Geometry check sheet. Reference: the model listing, model coordinates, mm. A direction names the side the tool comes from. Round coordinates to 2 decimals unless told otherwise and drop trailing zeros. Write each loop counter-clockwise with the first axis right and the second up, starting at its lowest first coordinate (ties: lowest second). Pieces come first, ordered by that corner, then holes. Notation, with made-up numbers: (24, 76.25) -> (74, 76.25) arc R25 ccw to (74, 97.25) -> close; hole circle Ø8 at (-8, 77). An arc over 180 degrees is marked (long way). One line per question, with ' | ' between items.
```python
from build123d import *

# Parameters (mm, degrees)
SKETCH_W           = 25.5
SKETCH_H           = 20.5
PAD_DEPTH          = 32
POCKET_DEPTH       = 20.501
SKETCH002_W        = 25.5
SKETCH002_H        = 2
POCKET001_DEPTH    = 2.1
SKETCH003_W        = 1.7
SKETCH003_H        = 9.5
POCKET002_DEPTH    = 12.5
SKETCH004_R        = 1.6
POCKET003_DEPTH    = 32.001
SKETCH005_R        = 3.6
POCKET004_DEPTH    = 2
SKETCH006_R        = 9
POCKET005_DEPTH    = 2
SKETCH007_R        = 3.6
POCKET006_DEPTH    = 19
SKETCH008_W        = 2.9999909846
SKETCH008_H        = 7.2
POCKET007_DEPTH    = 19
SKETCH009_W        = 2.9999856852
SKETCH009_H        = 3.2
POCKET008_DEPTH    = 7.5
SKETCH010_W        = 13
SKETCH010_H        = 15.5
PAD001_DEPTH       = 8.5
SKETCH011_W        = 16
SKETCH011_H        = 10
POCKET009_DEPTH    = 24
SKETCH012_W        = 4
SKETCH012_H        = 7.2
POCKET010_DEPTH    = 9
SKETCH013_W        = 1.5
SKETCH013_H        = 1.85
PAD002_DEPTH       = 15.5
PAD002_FACE36_W    = 4.15
PAD002_FACE36_H    = 10
POCKET011_DEPTH    = 1.5
SKETCH014_R        = 1.5
POCKET012_DEPTH    = 34.001
POCKET012_FACE43_W = 1.5
POCKET012_FACE43_H = 15.5
POCKET013_DEPTH    = 1.85
SKETCH015_W        = 4
SKETCH015_H        = 4.8
SKETCH015_H_2      = 3
POCKET014_DEPTH    = 2
POCKET015_DEPTH    = 8.5
PAD003_DEPTH       = 25
SKETCH018_W        = 1
SKETCH018_H        = 1
POCKET016_DEPTH    = 25
SKETCH019_W        = 2
SKETCH019_H        = 2
PAD004_DEPTH       = 10
SKETCH020_W        = 1
SKETCH020_H        = 2
PAD005_DEPTH       = 22.5
POCKET017_DEPTH    = 25
PAD006_DEPTH       = 25
PAD007_DEPTH       = 1
POCKET018_DEPTH    = 0.5
PAD008_DEPTH       = 58
POCKET019_DEPTH    = 5.851
PAD009_DEPTH       = 9.4
SKETCH024_R        = 1.5
PAD010_DEPTH       = 3


with BuildPart() as part:
    # Sketch → Pad (new body)
    with BuildSketch(Plane.XY):
        with Locations((12.75, 10.25)):
            Rectangle(SKETCH_W, SKETCH_H)
    extrude(amount=PAD_DEPTH)

    # Sketch001 (on Face1 of Pad) → Pocket (cut, through all)
    with BuildSketch(Plane.XZ):
        Polygon((0, 22), (23.5, 32), (0, 32), align=None)
    extrude(amount=-POCKET_DEPTH, mode=Mode.SUBTRACT)

    # Sketch002 (on Face1 of Pocket) → Pocket001 (cut)
    with BuildSketch(Plane.XZ):
        with Locations((12.75, 1)):
            Rectangle(SKETCH002_W, SKETCH002_H)
    extrude(amount=-POCKET001_DEPTH, mode=Mode.SUBTRACT)

    # Sketch003 (on Face1 of Pocket001) → Pocket002 (cut)
    with BuildSketch(Plane.XZ):
        with Locations((24.65, 4.75)):
            Rectangle(SKETCH003_W, SKETCH003_H)
    extrude(amount=-POCKET002_DEPTH, mode=Mode.SUBTRACT)

    # Sketch004 (on Face10 of Pocket002) → Pocket003 (cut, through all)
    with BuildSketch(Plane(origin=(0, 0, 0), x_dir=(1, 0, 0), z_dir=(0, 0, -1))):
        with Locations((4, -10.25)):
            Circle(SKETCH004_R)
        with Locations((22.5, -10.25)):
            Circle(SKETCH004_R)
    extrude(amount=-POCKET003_DEPTH, mode=Mode.SUBTRACT)

    # Sketch005 (on Face10 of Pocket003) → Pocket004 (cut)
    with BuildSketch(Plane(origin=(0, 0, 0), x_dir=(1, 0, 0), z_dir=(0, 0, -1))):
        with Locations((4, -10.25)):
            Circle(SKETCH005_R)
        with Locations((22.5, -10.25)):
            Circle(SKETCH005_R)
    extrude(amount=-POCKET004_DEPTH, mode=Mode.SUBTRACT)

    # Sketch006 (on Face10 of Pocket004) → Pocket005 (cut)
    with BuildSketch(Plane(origin=(0, 0, 0), x_dir=(1, 0, 0), z_dir=(0, 0, -1))):
        with Locations((13.25, -10.25)):
            Circle(SKETCH006_R)
    extrude(amount=-POCKET005_DEPTH, mode=Mode.SUBTRACT)

    # Sketch007 (on Face5 of Pocket005) → Pocket006 (cut)
    with BuildSketch(Plane.XY.offset(32)):
        with Locations((4, 10.25)):
            Circle(SKETCH007_R)
        with Locations((22.5, 10.25)):
            Circle(SKETCH007_R)
    extrude(amount=-POCKET006_DEPTH, mode=Mode.SUBTRACT)

    # Sketch008 (on Face5 of Pocket006) → Pocket007 (cut)
    with BuildSketch(Plane.XY.offset(32)):
        with Locations((24.0000045077, 10.25)):
            Rectangle(SKETCH008_W, SKETCH008_H)
    extrude(amount=-POCKET007_DEPTH, mode=Mode.SUBTRACT)

    # Sketch009 (on Face8 of Pocket007) → Pocket008 (cut)
    with BuildSketch(Plane(origin=(0, 0, 2), x_dir=(1, 0, 0), z_dir=(0, 0, -1))):
        with Locations((24.0000071574, -10.25)):
            Rectangle(SKETCH009_W, SKETCH009_H)
    extrude(amount=-POCKET008_DEPTH, mode=Mode.SUBTRACT)

    # Sketch010 (on Face3 of Pocket008) → Pad001 (join)
    with BuildSketch(Plane.YZ.offset(25.5)):
        with Locations((14, 24.25)):
            Rectangle(SKETCH010_W, SKETCH010_H)
    extrude(amount=PAD001_DEPTH)

    # Sketch011 (on Face7 of Pad001) → Pocket009 (cut)
    with BuildSketch(Plane(origin=(0, 0, 0), x_dir=(0, -1, 0), z_dir=(-1, 0, 0))):
        with Locations((-10, 27)):
            Rectangle(SKETCH011_W, SKETCH011_H)
    extrude(amount=-POCKET009_DEPTH, mode=Mode.SUBTRACT)

    # Sketch012 (on Face26 of Pocket009) → Pocket010 (cut)
    with BuildSketch(Plane.XY.offset(22)):
        with Locations((2, 10.25)):
            Rectangle(SKETCH012_W, SKETCH012_H)
    extrude(amount=-POCKET010_DEPTH, mode=Mode.SUBTRACT)

    # Sketch013 (on Face36 of Pocket010) → Pad002 (join)
    with BuildSketch(Plane.XY.offset(32)):
        with Locations((24.75, 7.575)):
            Rectangle(SKETCH013_W, SKETCH013_H)
    extrude(amount=-PAD002_DEPTH)

    # Pad002 Face36 → Pocket011 (cut)
    with BuildSketch(Plane(origin=(24, 15.925, 27), x_dir=(0, 1, 0), z_dir=(-1, 0, 0))):
        Rectangle(PAD002_FACE36_W, PAD002_FACE36_H)
    extrude(amount=-POCKET011_DEPTH, mode=Mode.SUBTRACT)

    # Sketch014 (on Face35 of Pocket011) → Pocket012 (cut, through all)
    with BuildSketch(Plane.YZ.offset(34)):
        with Locations((11, 26)):
            Circle(SKETCH014_R)
    extrude(amount=-POCKET012_DEPTH, mode=Mode.SUBTRACT)

    # Pocket012 Face43 → Pocket013 (cut)
    with BuildSketch(Plane(origin=(24.75, 8.5, 24.25), x_dir=(1, 0, 0), z_dir=(0, 1, 0))):
        Rectangle(POCKET012_FACE43_W, POCKET012_FACE43_H)
    extrude(amount=-POCKET013_DEPTH, mode=Mode.SUBTRACT)

    # Sketch015 (on Face2 of Pocket013) → Pocket014 (cut)
    with BuildSketch(Plane(origin=(0, 0, 0), x_dir=(1, 0, 0), z_dir=(0, 0, -1))):
        with Locations((13.25, -18.1)):
            Rectangle(SKETCH015_W, SKETCH015_H)
        with Locations((2, -10.25)):
            Rectangle(SKETCH015_W, SKETCH015_H_2)
    extrude(amount=-POCKET014_DEPTH, mode=Mode.SUBTRACT)

    # Sketch016 (on Face45 of Pocket014) → Pocket015 (cut)
    with BuildSketch(Plane.YZ.offset(34)):
        Polygon((13.85, 16.5), (20.5, 23.15), (20.5, 16.5), align=None)
    extrude(amount=-POCKET015_DEPTH, mode=Mode.SUBTRACT)

    # Sketch017 (on Face46 of Pocket015) → Pad003 (join)
    with BuildSketch(Plane.YZ.offset(34)):
        Polygon((20.5, 31), (14.5, 25), (14.5, 17.15), (20.5, 23.15), align=None)
    extrude(amount=PAD003_DEPTH)

    # Sketch018 (on Face53 of Pad003) → Pocket016 (cut)
    with BuildSketch(Plane.YZ.offset(59)):
        with Locations((20, 30.5)):
            Rectangle(SKETCH018_W, SKETCH018_H)
        with Locations((15, 17.65)):
            Rectangle(SKETCH018_W, SKETCH018_H)
    extrude(amount=-POCKET016_DEPTH, mode=Mode.SUBTRACT)

    # Sketch019 (on Face45 of Pocket016) → Pad004 (join)
    with BuildSketch(Plane.XY.offset(32)):
        with Locations((24.5, 17)):
            Rectangle(SKETCH019_W, SKETCH019_H)
    extrude(amount=-PAD004_DEPTH)

    # Sketch020 (on Face60 of Pad004) → Pad005 (join)
    with BuildSketch(Plane.XY.offset(32)):
        with Locations((26, 6.5)):
            Rectangle(SKETCH020_W, SKETCH020_H)
    extrude(amount=-PAD005_DEPTH)

    # Sketch021 (on Face46 of Pad005) → Pocket017 (cut)
    with BuildSketch(Plane.YZ.offset(59)):
        Polygon((14.5, 25), (18.425, 21.075), (14.5, 17.15), align=None)
    extrude(amount=-POCKET017_DEPTH, mode=Mode.SUBTRACT)

    # Sketch022 (on Face49 of Pocket017) → Pad006 (join)
    with BuildSketch(Plane.YZ.offset(59)):
        Polygon((18.425, 21.075), (17.425, 21.075), (17.425, 22.075), align=None)
    extrude(amount=-PAD006_DEPTH)

    # Pad006 Face64 → Pad007 (add)
    with BuildSketch(Plane(origin=(59, 18.28427215, 25.3924064799), x_dir=(0, -1, 0), z_dir=(1, 0, 0))):
        Polygon((-2.21572785, -4.6075935201), (-1.21572785, -4.6075935201), (3.78427215, 0.3924064799), (0.85927215, 3.3174064799), (0.85927215, 4.3174064799), (-0.14072785, 4.3174064799), (-2.21572785, 2.2424064799), align=None)
    extrude(amount=PAD007_DEPTH)

    # Pad007 Face4 → Pocket018 (cut)
    with BuildSketch(Plane(origin=(12.6211473302, 9.1246275662, 2), x_dir=(0, -1, 0), z_dir=(0, 0, -1))):
        with BuildLine():
            Line((0.3746275662, 12.6211473302), (-2.6253724338, 12.6211473302))
            Line((-2.6253724338, 12.6211473302), (-2.6253724338, 11.8937609646))
            ThreePointArc((-2.6253724338, 11.8937609646), (-4.3864646733, 10.1460333605), (-4.5985386893, 7.6739851681))
            ThreePointArc((-4.5985386893, 7.6739851681), (-8.0127244114, 5.1646249332), (-9.9003368212, 1.3711473302))
            Line((-9.9003368212, 1.3711473302), (-11.3753724338, 1.3711473302))
            Line((-11.3753724338, 1.3711473302), (-11.3753724338, -2.6288526698))
            Line((-11.3753724338, -2.6288526698), (-9.9003368212, -2.6288526698))
            ThreePointArc((-9.9003368212, -2.6288526698), (-8.0127244114, -6.4223302727), (-4.5985386893, -8.9316905076))
            ThreePointArc((-4.5985386893, -8.9316905076), (-4.5485570394, -10.9932166839), (-3.3753724338, -12.6891017691))
            Line((-3.3753724338, -12.6891017691), (-3.3753724338, -11.1788526698))
            Line((-3.3753724338, -11.1788526698), (-2.7253724338, -11.1788526698))
            Line((-2.7253724338, -11.1788526698), (-2.7253724338, -9.8788669846))
            ThreePointArc((-2.7253724337, -9.8788669846), (-2.71357708, -9.6849300003), (-2.6783614872, -9.4938526698))
            ThreePointArc((-2.6783614872, -9.4938526698), (-1.1253724338, -8.2788526698), (0.4276166196, -9.4938526698))
            ThreePointArc((0.4276166196, -9.4938526698), (0.4628322125, -9.6849300003), (0.4746275662, -9.8788669846))
            Line((0.4746275662, -9.8788669846), (0.4746275662, -11.1788526698))
            Line((0.4746275662, -11.1788526698), (2.2317096326, -11.1788526698))
            ThreePointArc((2.2317096326, -11.1788526698), (2.4698337467, -10.0645742886), (2.3477938218, -8.9316905076))
            ThreePointArc((2.3477938218, -8.9316905076), (5.1038193792, -7.124787503), (7.0246275662, -4.4469019099))
            Line((7.0246275662, -4.4469019099), (7.0246275662, -11.1788526698))
            Line((7.0246275662, -11.1788526698), (9.1246275662, -11.1788526698))
            Line((9.1246275662, -11.1788526698), (9.1246275662, 12.6211473302))
            Line((9.1246275662, 12.6211473302), (7.0246275662, 12.6211473302))
            Line((7.0246275662, 12.6211473302), (7.0246275662, 3.1891965703))
            ThreePointArc((7.0246275662, 3.1891965703), (5.1038193792, 5.8670821634), (2.3477938218, 7.6739851681))
            ThreePointArc((2.3477938218, 7.6739851681), (2.1357198057, 10.1460333605), (0.3746275662, 11.8937609646))
            Line((0.3746275662, 11.8937609646), (0.3746275662, 12.6211473302))
        make_face()
        with BuildLine():
            ThreePointArc((-2.6253724338, 9.1779237665), (-1.1253724338, 10.2211473302), (0.3746275662, 9.1779237665))
            ThreePointArc((0.3746275662, 9.1779237665), (0.4721009632, 8.7110291747), (0.4276166196, 8.2361473302))
            ThreePointArc((0.4276166196, 8.2361473302), (-0.1394718303, 7.3609886101), (-1.1253724338, 7.0211473302))
            ThreePointArc((-1.1253724338, 7.0211473302), (-2.1112730373, 7.3609886101), (-2.6783614872, 8.2361473302))
            ThreePointArc((-2.6783614872, 8.2361473302), (-2.7228458307, 8.7110291747), (-2.6253724338, 9.1779237665))
        make_face(mode=Mode.SUBTRACT)
    extrude(amount=-POCKET018_DEPTH, mode=Mode.SUBTRACT)

    # Sketch023 (on Face35 of Pocket018) → Pad008 (join)
    with BuildSketch(Plane.YZ.offset(60)):
        Polygon((20.5, 23.15), (26.35, 29), (26.35, 30), (20.5, 30), align=None)
    extrude(amount=-PAD008_DEPTH)

    # Pad008 Face47 → Pocket019 (cut, through all)
    with BuildSketch(Plane(origin=(7.6093987764, 20.5, 27.6250202352), x_dir=(-1, 0, 0), z_dir=(0, -1, 0))):
        Polygon((4.9068987764, 4.4750202352), (-11.1906012236, -2.3749797648), (5.6093987764, -2.3749797648), (5.6093987764, 4.4750202352), align=None)
    extrude(amount=-POCKET019_DEPTH, mode=Mode.SUBTRACT)

    # Pocket019 Face62 → Pad009 (add)
    with BuildSketch(Plane(origin=(60, 20.1386845476, 26.3510071585), x_dir=(0, -1, 0), z_dir=(1, 0, 0))):
        Polygon((1.7136845476, 5.2760071585), (-6.2113154524, -2.6489928415), (-6.2113154524, -3.6489928415), (0.6386845476, -3.6489928415), (5.6386845476, 1.3510071585), (2.7136845476, 4.2760071585), (2.7136845476, 5.2760071585), align=None)
    extrude(amount=PAD009_DEPTH)

    # Sketch024 (on Face60 of Pad009) → Pad010 (join)
    with BuildSketch(Plane.YZ.offset(69.4)):
        with BuildLine():
            ThreePointArc((11, 30), (7.30448187, 27.5307337295), (8.1715728753, 23.1715728753))
            Line((8.1715728753, 23.1715728753), (10.2681457504, 21.075))
            Line((18.425, 21.075), (10.2681457504, 21.075))
            Line((18.425, 21.075), (26.35, 29))
            Line((26.35, 29), (26.35, 30))
            Line((26.35, 30), (20.5, 30))
            Line((20.5, 30), (11, 30))
        make_face()
        with Locations((11, 26)):
            Circle(SKETCH024_R, mode=Mode.SUBTRACT)
    extrude(amount=PAD010_DEPTH)


solid = part.part
```
(1) Go/stop test with flat-tipped pins: pin 1 (1.1 mm diameter, centred on x = 55.5, z = 22, fed in from -Y); pin 2 (8 mm diameter, centred on x = 8.5, y = 9, fed in from +Z); pin 3 (5 mm diameter, centred on x = 47.5, z = 21, fed in from -Y); pin 4 (4 mm diameter, centred on y = 16.5, z = 4.5, fed in from -X). Record where each tip stops, or that it passes through.
Resolved:
pin 1: stops at y = 16.95 | pin 2: stops at z = 22 | pin 3: stops at y = 16 | pin 4: stops at x = 0
(2) Sectioned sample at B-B on z = 14.5. Record the cut outline in (x, y).
Resolved:
outline: (0, 0) -> (25.5, 0) -> (25.5, 5.5) -> (26.5, 5.5) -> (26.5, 7.5) -> (25.5, 7.5) -> (25.5, 6.65) -> (22.5, 6.65) arc R3.6 cw to (22.5, 13.85) -> (25.5, 13.85) -> (25.5, 20.5) -> (0, 20.5) -> (0, 13.85) -> (4, 13.85) arc R3.6 cw to (4, 6.65) -> (0, 6.65) -> close
(3) Access from +Z, -Z, +X, -X, +Y, -Y to the whole of each face (thin tool, end or side, straight path). Record for faces 1 (the flat face through (17, 18, 25)), 2 (the flat face through (30, 7.5, 24)), 3 (the flat face through (25, 12.5, 6)), 4 (the flat face through (25.5, 12.3, 24.7)), 5 (the flat face through (11.25, 20, 1)).
Resolved:
face 1: +Z, -X | face 2: +Z, -Z, -Y | face 3: -Z, +X, -Y | face 4: +Z | face 5: -Z, +Y, -Y
(4) Sectioned sample at C-C on z = 7.5. Record the cut outline in (x, y).
Resolved:
outline: (0, 0) -> (23.8, 0) -> (23.8, 8.65) -> (22.5, 8.65) arc R1.6 cw to (22.5, 11.85) -> (23.8, 11.85) -> (23.8, 12.5) -> (25.5, 12.5) -> (25.5, 20.5) -> (0, 20.5) -> close; hole circle Ø3.2 at (4, 10.25)
(5) Draft check along X on faces 6 (the cylindrical face through (2.443, 13.496, 1.232)), 7 (the cylindrical face through (70.88, 7.33, 27.59)), 8 (the flat face through (25.5, 17, 9)). Enter one of: +X half, -X half, draft (parallel to the pull), parting line (faces both ways), or undercut.
Resolved:
face 6: undercut | face 7: draft | face 8: +X half
(6) Sectioned sample at A-A on z = 26. Record the cut outline in (x, y).
Resolved:
outline: (9.4, 0) -> (25.5, 0) -> (25.5, 5.5) -> (26.5, 5.5) -> (26.5, 7.5) -> (34, 7.5) -> (34, 9.5) -> (25.5, 9.5) -> (25.5, 6.65) -> (24, 6.65) -> (24, 2) -> (9.4, 2) -> close; (9.4, 18) -> (23.5, 18) -> (23.5, 16) -> (25.5, 16) -> (25.5, 12.5) -> (34, 12.5) -> (34, 15.5) -> (69.4, 15.5) -> (69.4, 12.5) -> (72.4, 12.5) -> (72.4, 23.35) -> (9.4, 23.35) -> close; (69.4, 7) -> (72.4, 7) -> (72.4, 9.5) -> (69.4, 9.5) -> close
(7) Sectioned sample at D-D on y = 4.25. Record the cut outline in (x, z), then the cut area to 3 significant figures.
Resolved:
outline: (0, 0) -> (6.54, 0) -> (6.54, 2.5) -> (19.96, 2.5) -> (19.96, 0) -> (23.8, 0) -> (23.8, 9.5) -> (25.5, 9.5) -> (25.5, 32) -> (24, 32) -> (24, 22) -> (0, 22) -> close | area: 526 mm2
(8) Material ranges on line 1 (Z direction, x = 71.2, y = 11) (3 decimals); line 2 (Y direction, x = 22.5, z = 5.25); line 3 (X direction, y = 14.75, z = 25.5), recorded low to high.
Resolved:
line 1: z = 21.075 to 24.5, 27.5 to 30 | line 2: y = 0 to 8.65, 11.85 to 20.5 | line 3: x = 25.5 to 34, 69.4 to 72.4
